```python
from build123d import *

# Parameters (mm, degrees)
EXTRUDE_1_DEPTH = 10


with BuildPart() as part:
    # Эскиз1_fr → Бобышка-Вытянуть1 (new body)
    with BuildSketch(Plane.XY):
        with BuildLine():
            add(Edge.make_bspline(
                [(-97.969549234, -25.769768053), (-112.011160689, -25.769768053), (-131.292525164, -19.025155818), (-131.292525164, 0)],
                knots=[0, 0, 0, 0, 1, 1, 1, 1], degree=3))
            Line((-131.292525164, 0), (-131.292525164, 43.097715536))
            add(Edge.make_bspline(
                [(-103.301225383, 67.978870897), (-115.500001367, 70.63077872), (-131.292525164, 63.393306184), (-131.292525164, 43.097715536)],
                knots=[0, 0, 0, 0, 1, 1, 1, 1], degree=3))
            Line((-103.301225383, 67.978870897), (-41.986949672, 54.649680525))
            add(Edge.make_bspline(
                [(0, 20), (0, 38.146025899), (-14.209474182, 48.611098897), (-41.986949672, 54.649680525)],
                knots=[0, 0, 0, 0, 1, 1, 1, 1], degree=3))
            Line((0, 20), (0, 0))
            add(Edge.make_bspline(
                [(-33.545129103, -25.769768053), (-19.444866568, -25.769768053), (0, -19.063757455), (0, 0)],
                knots=[0, 0, 0, 0, 1, 1, 1, 1], degree=3))
            Line((-33.545129103, -25.769768053), (-97.969549234, -25.769768053))
        make_face()
        with BuildLine():
            ThreePointArc((-58.66509027, 40.632464429), (-56.891886772, 37.874147876), (-54.133570218, 39.647351375))
            Line((-54.133570218, 39.647351375), (-52.067053016, 49.153330507))
            ThreePointArc((-52.067053016, 49.153330507), (-53.840256514, 51.91164706), (-56.598573068, 50.138443562))
            Line((-56.598573068, 50.138443562), (-58.66509027, 40.632464429))
        make_face(mode=Mode.SUBTRACT)
    extrude(amount=EXTRUDE_1_DEPTH)


solid = part.part
```
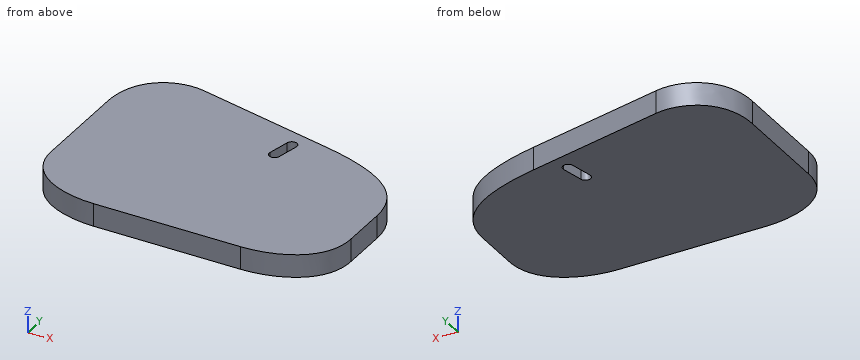
Design review of the part built by this model. Coordinates are the model's own, in mm. Give positions to 0.01 mm unless a question says otherwise; leave off trailing zeros. Order: outer loops, then holes, each group sorted by start corner. A loop starts at its lowest first (then second) coordinate and runs counter-clockwise, first axis right, second up. Notation, with made-up numbers: (21.25, -23.5) - (27.25, -23.5) arc R18 cw to (27.25, -2.5) - close; hole circle Ø2 at (86, 55.5). An arc over 180 degrees is marked (long way). Use a Markdown table: item, result. Add a question column.
(1) Add section A-A on x = -44. Give the boundary of the cut face in (y, z), then the cut area to 3 significant figures.
(2) Wall thickness on probe 1 along X at (y, z) = (-1, 3.25); probe 2 along X at (y, z) = (46, 1); probe 3 along X at (y, z) = (-8.5, 6.75): over which ranges is each line inside the solid? List them lowest first. Write a range as [from, to].
(3) Add section B-B on x = -87. Give the boundary of the cut face in (y, z).
(4) Clearance check with flat-ended pins moving along their axes: P1, Ø4, axis at x = -112.5, z = 3, coming from the -Y side; P2, Ø6, axis at y = 37, z = 6, coming from the +X side; P3, Ø5, axis at x = -42.5, z = 2, coming from the +Y side. State where each tip first meets the part, or that it passes through.
Report:
| question | item | result |
|---|---|---|
| 1 | outline | (-25.77, 0) - (55.09, 0) - (55.09, 10) - (-25.77, 10) - close |
| 1 | area | 809 mm² |
| 2 | probe 1 | x = [-131.27, -0.02] |
| 2 | probe 2 | x = [-131.18, -57.5], [-52.75, -16.82] |
| 2 | probe 3 | x = [-129.8, -1.49] |
| 3 | outline | (-25.77, 0) - (64.44, 0) - (64.44, 10) - (-25.77, 10) - close |
| 4 | P1 | stops at y = -24.05 |
| 4 | P2 | stops at x = -3.61 |
| 4 | P3 | stops at y = 55.3 |
